Check sheet for the drawn part. Datum: minimum x, y, z corner. Units: mm. A direction names the side the tool comes from. Give positions to 0.01 mm unless a question says otherwise; leave off trailing zeros. Order: outer loops, then holes, each group sorted by start corner. A loop starts at its lowest first (then second) coordinate and runs counter-clockwise, first axis right, second up. Notation, with made-up numbers: (71, 60) -> (115, 60) arc R21 ccw to (115, 92) -> close; hole circle Ø2 at (-39.5, 15). An arc over 180 degrees is marked (long way). Answer in a Markdown table with one row per item. Add a question column.
(1) Release check for a two-part mould opening along Y. For the marked faces 3 and 4 record: released by +Y, released by -Y, zero draft, split by the parting line, or undercut.
(2) Set-up check for the marked faces 1 and 2: record each of +Z, -Z, +X, -X, +Y, -Y from which the full face is reachable in a straight line by a thin tool's end or side.
(3) Cross-section at D-D (y = 1.5). Record the cut outline in (x, z).
(4) Thickness scan on L1, parallel to X at y = 7.5, z = 5.75; L2, parallel to X at y = 7, z = 7.75 (1 decimal); L3, parallel to X at y = 6, z = 11.5. Record the ranges inside material, lowest first. Write a range as [from, to].
(5) Go/stop test with flat-tipped pins: pin 1 (1.8 mm diameter, centred on x = 51.98, y = 7.5, fed in from -Z); pin 2 (6 mm diameter, centred on y = 8.5, z = 6.5, fed in from -X); pin 3 (6 mm diameter, centred on x = 25, z = 12, fed in from +Y); pin 4 (2 mm diameter, centred on x = 43.5, y = 6, fed in from +Z). Record where each tip stops, or that it passes through.
(6) Cross-section at A-A (y = 7.5). Record the cut outline in (x, z).
(7) Cross-section at C-C (x = 22.5). Record the cut outline in (y, z) (1 decimal), then the cut area to 3 significant figures.
(8) Cross-section at B-B (z = 6). Record the cut outline in (x, y).
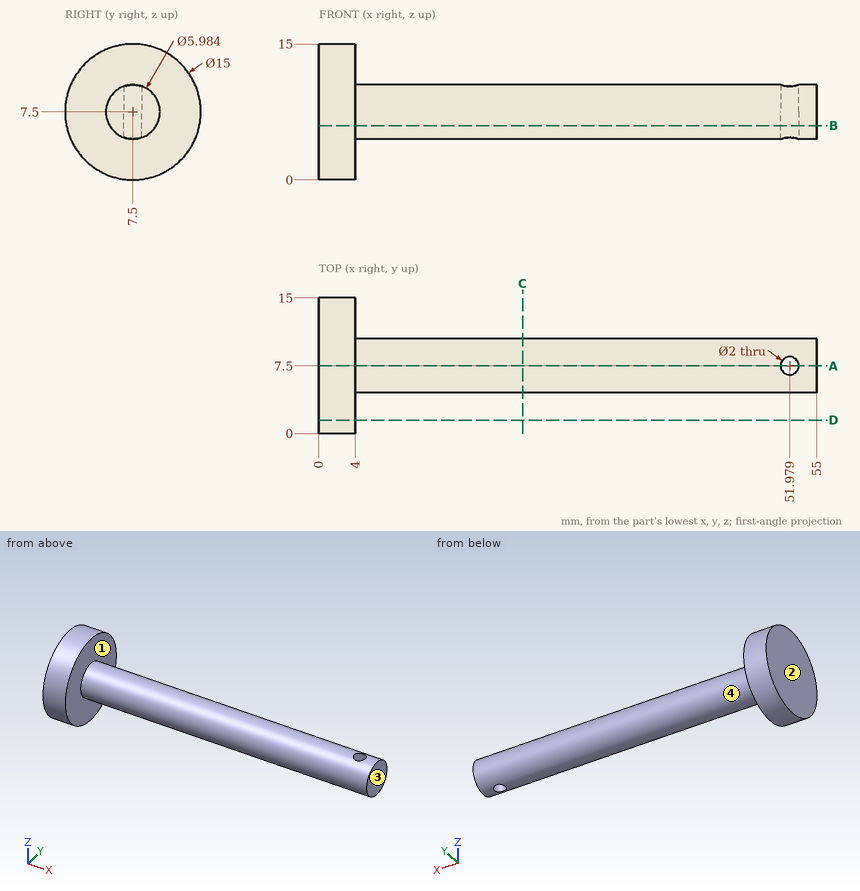
Answer below:
| question | item | result |
|---|---|---|
| 1 | face 3 | zero draft |
| 1 | face 4 | split by the parting line |
| 2 | face 1 | +X |
| 2 | face 2 | +Z, -Z, -X, +Y, -Y |
| 3 | outline | (0, 3) -> (4, 3) -> (4, 12) -> (0, 12) -> close |
| 4 | L1 | x = [0, 50.98], [52.98, 55] |
| 4 | L2 | x = [0, 51.1], [52.8, 55] |
| 4 | L3 | x = [0, 4] |
| 5 | pin 1 | passes through |
| 5 | pin 2 | stops at x = 0 |
| 5 | pin 3 | stops at y = 10.09 |
| 5 | pin 4 | stops at z = 10.45 |
| 6 | outline | (0, 0) -> (4, 0) -> (4, 4.51) -> (50.98, 4.51) -> (50.98, 10.49) -> (4, 10.49) -> (4, 15) -> (0, 15) -> close; (52.98, 4.51) -> (55, 4.51) -> (55, 10.49) -> (52.98, 10.49) -> close |
| 7 | outline | circle Ø6 at (7.5, 7.5) |
| 7 | area | 28.1 mm² |
| 8 | outline | (0, 0.15) -> (4, 0.15) -> (4, 4.91) -> (55, 4.91) -> (55, 10.09) -> (4, 10.09) -> (4, 14.85) -> (0, 14.85) -> close; hole circle Ø2 at (51.98, 7.5) |
